from build123d import *

# Parameters (mm, degrees)
SKETCH2_W           = 60
SKETCH2_H           = 35
BOSS_EXTRUDE1_DEPTH = 3
SKETCH3_W           = 5
SKETCH3_H           = 35
BOSS_EXTRUDE2_DEPTH = 10
SKETCH4_R           = 2
CUT_EXTRUDE1_DEPTH  = 64.294944506


with BuildPart() as part:
    # Sketch2 → Boss-Extrude1 (new body)
    with BuildSketch(Plane.XY):
        Rectangle(SKETCH2_W, SKETCH2_H)
    extrude(amount=BOSS_EXTRUDE1_DEPTH)

    # Sketch3 → Boss-Extrude2 (add)
    with BuildSketch(Plane(origin=(0, 0, 0), x_dir=(-1, 0, 0), z_dir=(0, 0, -1))):
        with Locations((-27.5, 0)):
            Rectangle(SKETCH3_W, SKETCH3_H)
        with Locations((27.5, 0)):
            Rectangle(SKETCH3_W, SKETCH3_H)
    extrude(amount=BOSS_EXTRUDE2_DEPTH)

    # Sketch4 → Cut-Extrude1 (cut, through all)
    with BuildSketch(Plane(origin=(30, 0, 0), x_dir=(0, 0, -1), z_dir=(1, 0, 0))):
        with Locations((5, 12.5)):
            Circle(SKETCH4_R)
        with Locations((5, -12.5)):
            Circle(SKETCH4_R)
    extrude(amount=-CUT_EXTRUDE1_DEPTH, mode=Mode.SUBTRACT)


solid = part.part
Read the model definition and answer for the solid it produces. Units are mm, in the model's axes. A direction names the side the tool comes from. Coordinates: 2 decimals unless noted, no trailing zeros. Write each loop counter-clockwise with the first axis right and the second up, starting at its lowest first coordinate (ties: lowest second). Pieces come first, ordered by that corner, then holes. Notation, with made-up numbers: (1, 80) - (6, 80) arc R12 cw to (6, 94) - close; hole circle Ø6 at (33.5, 4). An arc over 180 degrees is marked (long way). One line per question, with ' | ' between items.
Q1. This flat-tipped pin is pushed along its axis until it touches: P1, Ø10.5, axis at x = -0.5, y = -7.5, coming from the -Z side. Where does it stop, or does it pass through?
Result set:
P1: z = 0
Q2. Determine the mould class of faces 1 (the cylindrical face through (-27.465, -11.148, -3.526)), 2 (the cylindrical face through (-27.465, 13.852, -3.526)), 3 (the flat face through (25, 0, -5)), 4 (the flat face through (0, 0, 0)) for opening direction Z: +Z half, -Z half, draft (parallel to the pull), parting line (faces both ways), or undercut.
Result set:
face 1: undercut | face 2: undercut | face 3: draft | face 4: -Z half
Q3. For faces 5 (the cylindrical face through (27.535, -11.148, -3.526)), 6 (the flat face through (-25, 0, -5)), determine the directions among +Z, -Z, +X, -X, +Y, -Y from which every point of the face is accessible in a straight line to the end or side of a thin tool.
Result set:
face 5: +X, -X | face 6: -Z, +Y, -Y
Q4. Find section B-B, the plane z = -5. Write down the section's boundary in (x, y).
Result set:
outline: (-30, -17.5) - (-25, -17.5) - (-25, -14.5) - (-30, -14.5) - close; (-30, -10.5) - (-25, -10.5) - (-25, 10.5) - (-30, 10.5) - close; (-30, 14.5) - (-25, 14.5) - (-25, 17.5) - (-30, 17.5) - close; (25, -17.5) - (30, -17.5) - (30, -14.5) - (25, -14.5) - close; (25, -10.5) - (30, -10.5) - (30, 10.5) - (25, 10.5) - close; (25, 14.5) - (30, 14.5) - (30, 17.5) - (25, 17.5) - close
Q5. Find section A-A, the plane y = 12.5. Write down the section's boundary in (x, z).
Result set:
outline: (-30, -10) - (-25, -10) - (-25, -7) - (-30, -7) - close; (-30, -3) - (-25, -3) - (-25, 0) - (25, 0) - (25, -3) - (30, -3) - (30, 3) - (-30, 3) - close; (25, -10) - (30, -10) - (30, -7) - (25, -7) - close
Q6. Find section C-C, the plane y = -1. Write down the section's boundary in (x, z).
Result set:
outline: (-30, -10) - (-25, -10) - (-25, 0) - (25, 0) - (25, -10) - (30, -10) - (30, 3) - (-30, 3) - close
Q7. Consider L1, parallel to Y at x = 28.35, z = -5; L2, parallel to X at y = -11.5, z = -3; L3, parallel to Z at x = -14.5, y = -16. Determine where each line is inside the solid, lowest interval first. Write a range as [from, to].
Result set:
L1: [-17.5, -14.5], [-10.5, 10.5], [14.5, 17.5] | L2: [-30, -25], [25, 30] | L3: [0, 3]
Q8. Find section D-D, the plane x = 3.5. Write down the section's boundary in (y, z), plus the area to 3 significant figures.
Result set:
outline: (-17.5, 0) - (17.5, 0) - (17.5, 3) - (-17.5, 3) - close | area: 105 mm^2
